Model file for the job. Use its own axes, mm. Face numbers are marked on the shaded views. A direction names the side the tool comes from. Coordinates: 2 decimals unless noted, no trailing zeros. Order: outer loops, then holes, each group sorted by start corner. A loop starts at its lowest first (then second) coordinate and runs counter-clockwise, first axis right, second up. Notation, with made-up numbers: (9, -30) -> (50, -30) arc R16 cw to (50, -20) -> close; hole circle Ø3 at (61.5, -26.5). An arc over 180 degrees is marked (long way). Return JSON: item names as keys, results as strings. Group by question number.
1) Pull direction Y, two halves, no side cores. Call the marked faces 6, 7 and 8: +Y half, -Y half, draft (parallel to the pull), parting line (faces both ways), or undercut.
2) Cut at A-A (y = 5.5). Write the cut outline in (x, z).
3) Probe line 1 (Z direction, x = 0, y = 8); line 2 (X direction, y = 4.25, z = 2); line 3 (X direction, y = 8, z = 4). List the from-to ranges inside material, lowest first.
4) Cut at B-B (z = 5). Write the cut outline in (x, y), and give its area (3 significant figures).
5) Cut at D-D (z = 0). Write the cut outline in (x, y), and give its area (3 significant figures).
6) Which spindle directions (+Z, -Z, +X, -X, +Y, -Y) get a long thin tool onto all of the face, cutting with end or side? Do the marked faces 1, 2, 3, 4 and 5. Say none if no direction does.
7) Flat gauge pins, fed straight in: pin 1 (9 mm diameter, centred on x = 54.29, z = 0.01, fed in from +Y); pin 2 (6 mm diameter, centred on x = 27.5, y = 7, fed in from -Z); pin 3 (3.5 mm diameter, centred on x = 30, y = 4, fed in from +Z). Where does each tip first touch, or does it go through?
8) Cut at C-C (x = 21.5). Write the cut outline in (y, z), and give its area (3 significant figures).
from build123d import *

# Parameters (mm, degrees)
SKETCH1_R               = 8.35
SKETCH1_R_2             = 4
BOSS_EXTRUDE1_DEPTH     = 12
CUT_EXTRUDE1_DEPTH      = 70.17162349
SKETCH4_R               = 3
CUT_EXTRUDE3_DEPTH      = 70.17162349
FILLET2_R               = 5
CUT_EXTRUDE4_DEPTH      = 67.593644564
CUT_EXTRUDE4_DEPTH_BACK = 67.593644564


with BuildPart() as part:
    # Sketch1 → Boss-Extrude1 (new body)
    with BuildSketch(Plane(origin=(0, 0, 0), x_dir=(1, 0, 0), z_dir=(0, 1, 0))):
        with BuildLine():
            Line((9.287087811, 10), (54.287087811, 10))
            ThreePointArc((54.287087811, 10), (64.293438841, 0.343976386), (55, -10))
            Line((55, -10), (9.287087811, -10))
            ThreePointArc((9.287087811, -10), (7.727462076, -10.20624754), (6.275059331, -10.810810811))
            ThreePointArc((6.275059331, -10.810810811), (-12.5, 0), (6.275059331, 10.810810811))
            ThreePointArc((6.275059331, 10.810810811), (7.727462076, 10.20624754), (9.287087811, 10))
        make_face()
        with Locations(Location((0, 0, 0), (0, 0, 270))):
            Circle(SKETCH1_R, mode=Mode.SUBTRACT)
        with Locations(Location((54.287087811, -0.012706095, 0), (0, 0, 270))):
            Circle(SKETCH1_R_2, mode=Mode.SUBTRACT)
    extrude(amount=BOSS_EXTRUDE1_DEPTH)

    # Sketch2 → Cut-Extrude1 (cut, through all)
    with BuildSketch(Plane.XY.offset(10)):
        Polygon((19.299793905, 12), (24.299793905, 7), (64.299793905, 7), (64.299793905, 12), align=None)
    extrude(amount=-CUT_EXTRUDE1_DEPTH, mode=Mode.SUBTRACT)

    # Sketch4 → Cut-Extrude3 (cut, through all)
    with BuildSketch(Plane.XY.offset(10)):
        with Locations((15.287087811, 5.5)):
            Circle(SKETCH4_R)
    extrude(amount=-CUT_EXTRUDE3_DEPTH, mode=Mode.SUBTRACT)

    # Fillet2
    fillet2_edges = [part.edges().sort_by_distance(p)[0] for p in [
        (24.299793905, 7, 0),
        (19.299793905, 12, 0),
    ]]
    fillet(fillet2_edges, radius=FILLET2_R)

    # Sketch5 → Cut-Extrude4 (cut, two sides: drawn at the far end of the back side and taken through both)
    with BuildSketch(Plane(origin=(0, 12, 0), x_dir=(1, 0, 0), z_dir=(0, 1, 0)).offset(-CUT_EXTRUDE4_DEPTH_BACK)):
        with BuildLine():
            Line((0, -3.5), (40, -3.5))
            ThreePointArc((40, -3.5), (43.5, 0), (40, 3.5))
            Line((40, 3.5), (0, 3.5))
            Line((0, 3.5), (0, -3.5))
        make_face()
    extrude(amount=CUT_EXTRUDE4_DEPTH + CUT_EXTRUDE4_DEPTH_BACK, mode=Mode.SUBTRACT)


solid = part.part
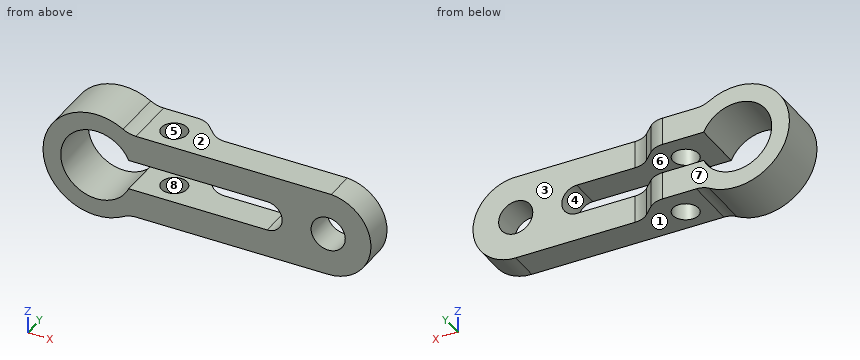
Answers below:
{
 "1": {"face 6": "draft", "face 7": "+Y half", "face 8": "undercut"},
 "2": {"outline": "(6.28, -10.81) arc R6 cw to (9.29, -10) -> (12.29, -10) -> (12.29, -3.5) -> (7.58, -3.5) arc R8.35 cw (long way) to (7.58, 3.5) -> (12.29, 3.5) -> (12.29, 10) -> (9.29, 10) arc R6 cw to (6.28, 10.81) arc R12.5 ccw (long way) to start; (18.29, -10) -> (54.29, -10) arc R10.01 ccw to (55, 10) -> (18.29, 10) -> (18.29, 3.5) -> (40, 3.5) arc R3.5 cw to (40, -3.5) -> (18.29, -3.5) -> close; hole circle Ø8 at (54.29, 0.01)"},
 "3": {"line 1": "z = -12.5 to -8.35, 8.35 to 12.5", "line 2": "x = -12.34 to -8.11, 42.87 to 50.82, 57.76 to 64.1", "line 3": "x = -11.84 to -7.33, 7.33 to 13.63, 16.95 to 23.37"},
 "4": {"outline": "(-11.46, 0) -> (-6.69, 0) -> (-6.69, 12) -> (-11.46, 12) -> close; (6.69, 0) -> (62.97, 0) -> (62.97, 7) -> (26.37, 7) arc R5 cw to (22.84, 8.46) -> (20.76, 10.54) arc R5 ccw to (17.23, 12) -> (6.69, 12) -> close; hole circle Ø6 at (15.29, 5.5)", "area": "498 mm^2"},
 "5": {"outline": "(-12.5, 0) -> (-8.35, 0) -> (-8.35, 12) -> (-12.5, 12) -> close; (43.5, 0) -> (50.29, 0) -> (50.29, 7) -> (43.5, 7) -> close; (58.29, 0) -> (64.3, 0) -> (64.3, 7) -> (58.29, 7) -> close", "area": "139 mm^2"},
 "6": {"face 1": "-Z, +X, +Y, -Y", "face 2": "+Z, +X, +Y, -Y", "face 3": "+Z, -Z, +X, +Y", "face 4": "+Y, -Y", "face 5": "+Z, -Z"},
 "7": {"pin 1": "stops at y = 7", "pin 2": "stops at z = -10", "pin 3": "stops at z = 10"},
 "8": {"outline": "(0, -10) -> (9.8, -10) -> (9.8, -3.5) -> (0, -3.5) -> close; (0, 3.5) -> (9.8, 3.5) -> (9.8, 10) -> (0, 10) -> close", "area": "127 mm^2"}
}
